Could you check a few things on this model? Use its own coordinates, in mm. Coordinates: 2 decimals unless noted, no trailing zeros. Write each loop counter-clockwise with the first axis right and the second up, starting at its lowest first coordinate (ties: lowest second). Pieces come first, ordered by that corner, then holes. Notation, with made-up numbers: M 80,-13 L 109,-13 A34 ccw 109,19 Z; hole C 48,10 d6. An arc over 180 degrees is marked long. Answer as CSV lines item,"result". Start each with the question number.
Item 1: I'm going to push flat-ended pins straight in: P1, Ø8, axis at x = 15, y = -13, coming from the -Z side; P2, Ø10, axis at x = 3.5, y = 10, coming from the +Z side. Where does each tip first touch, or does it pass through?
Item 2: Suppose I cut it at C-C, the plane z = 440. Write out the boundary of the cut face in (x, y) (3 decimals), and give its area (3 significant figures).
Item 3: If I drill on line 1 along Y through (x, z) = (-14.5, 283) (3 decimals), over which ranges is the centre line in solid material (lowest first)? Write a range as [from, to].
Item 4: Suppose I cut it at A-A, the plane x = 0.5. Write out the boundary of the cut face in (y, z) (3 decimals), and give its area (3 significant figures).
Autodesk Inventor part; units mm, degrees
ref_plane "Start Plane" through (0, 0, -19.05) normal (0, 0, 1) x (1, 0, 0)
ref_plane "End Plane" through (0, 0, 781.05) normal (0, 0, 1) x (1, 0, 0)
ref_plane "Work Plane5" through (0, 12.7, 781.05) normal (0, 0, 1) x (1, 0, 0)
ref_plane "Start Plane" through (0, 0, -19.05) normal (0, 0, 1) x (1, 0, 0)
ref_plane "End Plane" through (0, 0, 781.05) normal (0, 0, 1) x (1, 0, 0)
sketch "Sketch" plane through (0, 0, 0) normal (0, 0, 1) x (1, 0, 0)
  line L0 (-19.05, 19.05) -> (19.05, 19.05)
  line L1 (19.05, 19.05) -> (19.05, -19.05)
  line L2 (19.05, -19.05) -> (-19.05, -19.05)
  line L3 (-19.05, -19.05) -> (-19.05, 19.05)
  line L4 (15.875, 15.875) -> (-15.875, 15.875)
  line L5 (-15.875, 15.875) -> (-15.875, -15.875)
  line L6 (-15.875, -15.875) -> (15.875, -15.875)
  line L7 (15.875, -15.875) -> (15.875, 15.875)
  point P0 (0, 0)
  point P1 (0, 19.05)
  point P2 (-19.05, 0)
  dimension "width" = 38.1
  dimension "d1" = 3.175
extrude "Body" add sketch "Sketch" along normal up to surface (800.1 mm away) from surface at -19.05
sketch "Sketch4" plane through (0, 0, 0) normal (0, 0, 1) x (1, 0, 0)
  line L0 (0, 0) -> (10, 0)
ref_plane "Work Plane4" through (0, 0, 0) normal (0, -1, 0) x (1, 0, 0)
sketch "Sketch5" plane through (0, 0, 0) normal (0, -1, 0) x (1, 0, 0)
  line L0 (-2, -19.05) -> (12, -19.05)
  line L1 (-2, 781.05) -> (12, 781.05)
  dimension "d9" = 800.1
ref_plane "Work Plane5" through (0, 12.7, 781.05) normal (0, 0, 1) x (1, 0, 0)
split "Split1" plane through (0, 12.7, 781.05) removes the side toward (0, 0, 1)
ref_plane "Work Plane6" through (0, -12.7, -19.05) normal (0, 0, -1) x (-1, 0, 0)
split "Split2" plane through (0, -12.7, -19.05) removes the side toward (0, 0, -1)
equation "\"G_OFFSET_START\" = 19.05"
equation "\"G_OFFSET_END\" = 19.05"
equation "\"d4\" = -G_OFFSET_START"
equation "\"d5\" = length + G_OFFSET_END"
equation "\"G_L\" = 762"
properties part number "1.5x1.5x.125 Tube" material "Aluminum-6061"
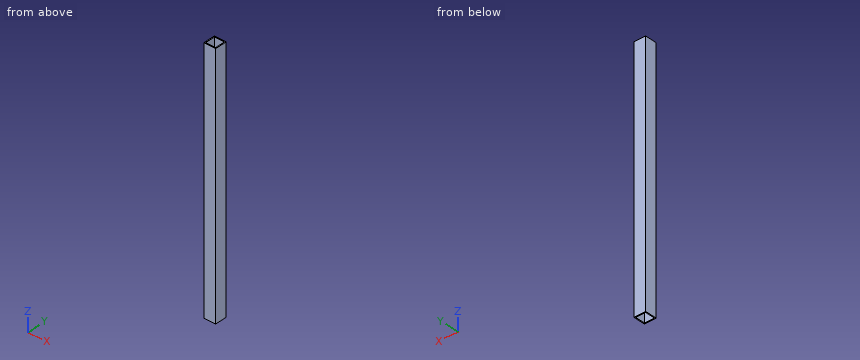
Ans:
1,P1,"stops at z = -19.05"
1,P2,"passes through"
2,outline,"M -19.05,-19.05 L 19.05,-19.05 L 19.05,19.05 L -19.05,19.05 Z; hole M -15.875,-15.875 L 15.875,-15.875 L 15.875,15.875 L -15.875,15.875 Z"
2,area,"444 mm^2"
3,line 1,"y = [-19.05, -15.875], [15.875, 19.05]"
4,outline,"M -19.05,-19.05 L -15.875,-19.05 L -15.875,781.05 L -19.05,781.05 Z; M 15.875,-19.05 L 19.05,-19.05 L 19.05,781.05 L 15.875,781.05 Z"
4,area,"5,080 mm^2"
